from build123d import *

# Parameters (mm, degrees)
BASE_FLANGE1_DEPTH           = 1.2192
EDGE_FLANGE1_STRIP_W         = 7.4168
EDGE_FLANGE1_STRIP_H         = 1.2192
EDGE_FLANGE1_STRIP_CUT_DEPTH = 203.2
EDGE_FLANGE1_DEPTH           = 203.2
EDGE_FLANGE2_STRIP_W         = 7.4168
EDGE_FLANGE2_STRIP_H         = 1.2192
EDGE_FLANGE2_STRIP_CUT_DEPTH = 302.3108
EDGE_FLANGE2_DEPTH           = 302.3108
F_1_4_0_25_DIAMETER_HOLE1_D  = 6.7564
SKETCH15_W                   = 152.4
SKETCH15_H                   = 44.45
CUT_EXTRUDE2_DEPTH           = 373.975962979
F_1_4_0_25_DIAMETER_HOLE3_D  = 6.7564
EDGE_FLANGE3_STRIP_W         = 7.4168
EDGE_FLANGE3_STRIP_H         = 1.2192
EDGE_FLANGE3_STRIP_CUT_DEPTH = 99.1108
EDGE_FLANGE3_DEPTH           = 99.1108


# Sheet-metal steps are written as plain solids
with BuildPart() as part:
    # Sketch1 → Base-Flange1 (new body)
    with BuildSketch(Plane(origin=(0, 0, 0), x_dir=(1, 0, 0), z_dir=(0, 1, 0))):
        Polygon((0, 0), (0, 203.2), (304.8, 203.2), (304.8, 127), (101.6, 127), (101.6, 0), align=None)
    extrude(amount=-BASE_FLANGE1_DEPTH)

    # Edge-Flange1 strip (across the edge) → Edge-Flange1 strip cut (cut)
    with BuildSketch(Plane.XY.offset(-203.2)):
        with Locations((-1.2192, -0.6096)):
            Rectangle(EDGE_FLANGE1_STRIP_W, EDGE_FLANGE1_STRIP_H)
    extrude(amount=EDGE_FLANGE1_STRIP_CUT_DEPTH, mode=Mode.SUBTRACT)

    # Edge-Flange1 section (across the edge) → Edge-Flange1 (add)
    with BuildSketch(Plane.XY.offset(-203.2)):
        with BuildLine():
            Line((0, 1.27), (0, 74.9808))
            Line((0, 74.9808), (1.2192, 74.9808))
            Line((1.2192, 74.9808), (1.2192, 1.27))
            ThreePointArc((1.2192, 1.27), (1.591174388, 0.371974388), (2.4892, 0))
            Line((2.4892, 0), (2.4892, -1.2192))
            ThreePointArc((2.4892, -1.2192), (0.7290698, -0.4901302), (0, 1.27))
        make_face()
    extrude(amount=EDGE_FLANGE1_DEPTH)

    # Edge-Flange2 strip (across the edge) → Edge-Flange2 strip cut (cut)
    with BuildSketch(Plane(origin=(304.8, 0, -203.2), x_dir=(0, 0, 1), z_dir=(-1, 0, 0))):
        with Locations((-1.2192, -0.6096)):
            Rectangle(EDGE_FLANGE2_STRIP_W, EDGE_FLANGE2_STRIP_H)
    extrude(amount=EDGE_FLANGE2_STRIP_CUT_DEPTH, mode=Mode.SUBTRACT)

    # Edge-Flange2 section (across the edge) → Edge-Flange2 (add)
    with BuildSketch(Plane(origin=(304.8, 0, -203.2), x_dir=(0, 0, 1), z_dir=(-1, 0, 0))):
        with BuildLine():
            Line((0, 1.27), (0, 75.229826743))
            Line((0, 75.229826743), (1.2192, 75.229826743))
            Line((1.2192, 75.229826743), (1.2192, 1.27))
            ThreePointArc((1.2192, 1.27), (1.591174388, 0.371974388), (2.4892, 0))
            Line((2.4892, 0), (2.4892, -1.2192))
            ThreePointArc((2.4892, -1.2192), (0.7290698, -0.4901302), (0, 1.27))
        make_face()
    extrude(amount=EDGE_FLANGE2_DEPTH)

    # 1/4 (0.25) Diameter Hole1 (through all)
    with Locations(Plane(origin=(74.174301672, 24.429826743, -203.2), x_dir=(0, -1, 0), z_dir=(0, 0, -1))):
        with Locations((0, 0)):
            Hole(F_1_4_0_25_DIAMETER_HOLE1_D / 2)

    # Sketch15 → Cut-Extrude2 (cut, through all)
    with BuildSketch(Plane(origin=(1.2192, 0, 0), x_dir=(0, 0, -1), z_dir=(1, 0, 0))):
        with Locations((76.2, 52.7558)):
            Rectangle(SKETCH15_W, SKETCH15_H)
    extrude(amount=-CUT_EXTRUDE2_DEPTH, mode=Mode.SUBTRACT)

    # 1/4 (0.25) Diameter Hole3 (through all)
    with Locations(Plane(origin=(199.080372839, 24.429826743, -203.2), x_dir=(0, -1, 0), z_dir=(0, 0, -1))):
        with Locations((0, 0)):
            Hole(F_1_4_0_25_DIAMETER_HOLE3_D / 2)

    # Edge-Flange3 strip (across the edge) → Edge-Flange3 strip cut (cut)
    with BuildSketch(Plane(origin=(2.4892, 0, 0), x_dir=(0, 0, -1), z_dir=(1, 0, 0))):
        with Locations((-1.2192, -0.6096)):
            Rectangle(EDGE_FLANGE3_STRIP_W, EDGE_FLANGE3_STRIP_H)
    extrude(amount=EDGE_FLANGE3_STRIP_CUT_DEPTH, mode=Mode.SUBTRACT)

    # Edge-Flange3 section (across the edge) → Edge-Flange3 (add)
    with BuildSketch(Plane(origin=(2.4892, 0, 0), x_dir=(0, 0, -1), z_dir=(1, 0, 0))):
        with BuildLine():
            Line((0, 1.27), (0, 24.1808))
            Line((0, 24.1808), (1.2192, 24.1808))
            Line((1.2192, 24.1808), (1.2192, 1.27))
            ThreePointArc((1.2192, 1.27), (1.591174388, 0.371974388), (2.4892, 0))
            Line((2.4892, 0), (2.4892, -1.2192))
            ThreePointArc((2.4892, -1.2192), (0.7290698, -0.4901302), (0, 1.27))
        make_face()
    extrude(amount=EDGE_FLANGE3_DEPTH)


solid = part.part
Part model, mm, in its own coordinate system. A direction names the side the tool comes from. Round coordinates to 2 decimals unless told otherwise and drop trailing zeros. Order: outer loops, then holes, each group sorted by start corner. A loop starts at its lowest first (then second) coordinate and runs counter-clockwise, first axis right, second up. Notation, with made-up numbers: (74, -24.75) -> (101, -24.75) arc R25 cw to (101, 3.25) -> close; hole circle Ø9 at (-12, 63.5). An arc over 180 degrees is marked (long way). Put each result on its own line as item: value.
Q1. Band-saw the part on A-A (y = 14.5). Give the cut face in (x, z).
From the geometry:
outline: (0, -203.2) -> (1.22, -203.2) -> (1.22, 0) -> (0, 0) -> close; (2.49, -203.2) -> (304.8, -203.2) -> (304.8, -201.98) -> (2.49, -201.98) -> close; (2.49, -1.22) -> (101.6, -1.22) -> (101.6, 0) -> (2.49, 0) -> close
Q2. Band-saw the part on C-C (z = -51). Give the cut face in (x, y).
From the geometry:
outline: (0, 1.27) arc R2.49 ccw to (2.49, -1.22) -> (101.6, -1.22) -> (101.6, 0) -> (2.49, 0) arc R1.27 cw to (1.22, 1.27) -> (1.22, 30.53) -> (0, 30.53) -> close
Q3. Band-saw the part on D-D (y = 43). Give the cut face in (x, z), and give its area (3 significant figures).
From the geometry:
outline: (0, -203.2) -> (1.22, -203.2) -> (1.22, -152.4) -> (0, -152.4) -> close; (2.49, -203.2) -> (304.8, -203.2) -> (304.8, -201.98) -> (2.49, -201.98) -> close
area: 431 mm2
Q4. Wall check: line 1 (Z direction, x = 97, y = 68); line 2 (Y direction, x = 102, z = -140.5); line 3 (X direction, y = 18.5, z = -76.5). Give the ranges that are in metal, low to high. Write a range as [from, to].
From the geometry:
line 1: z = [-203.2, -201.98]
line 2: y = [-1.22, 0]
line 3: x = [0, 1.22]
Q5. Tool access for faces 5 (the face through (101.6, -1, -64)), 6 (the face through (122, -1.219, -147)), 7 (the face through (122, 0, -147)): list every direction of +Z, -Z, +X, -X, +Y, -Y with a clear straight run to the whole face (end or side of a thin tool).
From the geometry:
face 5: +Z, +X, +Y, -Y
face 6: +Z, -Z, +X, -X, -Y
face 7: +X, +Y
Q6. Band-saw the part on B-B (x = 116). Give the cut face in (y, z), and give its area (3 significant figures).
From the geometry:
outline: (-1.22, -200.71) arc R2.49 ccw to (1.27, -203.2) -> (75.23, -203.2) -> (75.23, -201.98) -> (1.27, -201.98) arc R1.27 cw to (0, -200.71) -> (0, -127) -> (-1.22, -127) -> close
area: 184 mm2
Q7. Pull direction Z, two halves, no side cores. Call faces 1 (the face through (51, 13, 0)), 2 (the face through (51, 13, -1.219)), 3 (the face through (77.472, 23.697, -202.582)), 4 (the face through (156, 38, -203.2)): pulls with the +Z half, pulls with the -Z half, needs draft (parallel to the pull), parting line crosses it, or undercut.
From the geometry:
face 1: pulls with the +Z half
face 2: undercut
face 3: needs draft
face 4: pulls with the -Z half
Q8. Pin check, flat tips, straight feed: pin 1 Ø1.3 at (y, z) = (-0.5, -1.5) entering from +X; pin 2 Ø22 at (x, y) = (79, 53.5) entering from +Z; pin 3 Ø1 at (x, z) = (1, -185.5) entering from +Y. Stop position of each tip, or through.
From the geometry:
pin 1: stops at x = 101.6
pin 2: stops at z = -201.98
pin 3: stops at y = 74.98
